For this review, use the dimensioned drawing (mm, ordinates from the lowest corner) and the shaded views. A direction names the side the tool comes from. Round coordinates to 2 decimals unless told otherwise and drop trailing zeros. Loops run counter-clockwise (first coordinate to the right, second up) from the corner with the lowest first, then second, coordinate; pieces in that order, holes last. Notation, with made-up numbers: (50, -13.5) -> (89, -13.5) arc R30 cw to (89, 23.5) -> close; hole circle Ø6 at (63.5, 39.25). An arc over 180 degrees is marked (long way). Write each question's results on one line, items separated by ' | '.
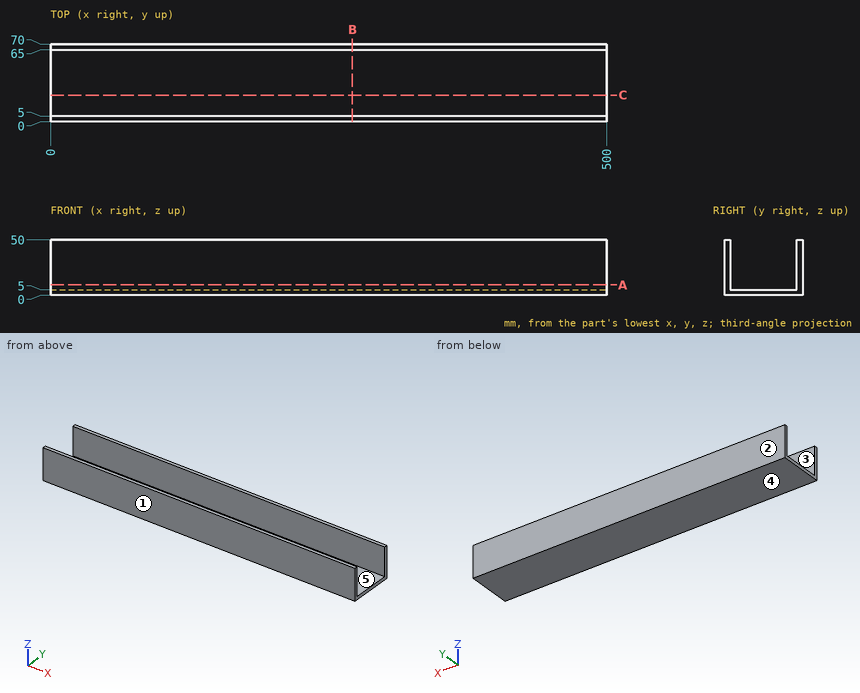
1. To check wall thickness, follow probe 1 along Y at (x, z) = (218, 17); probe 2 along Z at (x, y) = (90, 38). State the ranges of each line that lie inside material, in increasing order.
Values found:
probe 1: y = 0 to 5, 65 to 70 | probe 2: z = 0 to 5
2. Consider section C-C (y = 24). State the section outline as (x, z) points.
Values found:
outline: (0, 0) -> (500, 0) -> (500, 5) -> (0, 5) -> close
3. Draft analysis for pull direction Y (two halves, no side actions). For the marked faces 1, 2 and 3, state which applies: released by +Y, released by -Y, zero draft, split by the parting line, or undercut.
Values found:
face 1: released by -Y | face 2: released by +Y | face 3: undercut
4. Consider section A-A (z = 9.5). State the section outline as (x, y) points, plus the area to 3 significant figures.
Values found:
outline: (0, 0) -> (500, 0) -> (500, 5) -> (0, 5) -> close; (0, 65) -> (500, 65) -> (500, 70) -> (0, 70) -> close | area: 5,000 mm2
5. For pin 1 (5 mm diameter, centred on x = 345, y = 45, fed in from +Z), flat-tipped, find the tip position at first contact; note if it passes through.
Values found:
pin 1: stops at z = 5
6. Tool access review of the marked faces 4 and 5: name each direction out of +Z, -Z, +X, -X, +Y, -Y from which nothing blocks a thin tool from reaching the whole face with its end or side.
Values found:
face 4: -Z, +X, -X, +Y, -Y | face 5: +Z, +X, -X
7. Consider section B-B (x = 271.5). State the section outline as (y, z) points, plus the area to 3 significant figures.
Values found:
outline: (0, 0) -> (70, 0) -> (70, 50) -> (65, 50) -> (65, 5) -> (5, 5) -> (5, 50) -> (0, 50) -> close | area: 800 mm2
